Verification items for the finished model (mm, model axes). A direction names the side the tool comes from. Coordinates: 2 decimals unless noted, no trailing zeros. Order: outer loops, then holes, each group sorted by start corner. A loop starts at its lowest first (then second) coordinate and runs counter-clockwise, first axis right, second up. Notation, with made-up numbers: M -8,9 L 31,9 A28 ccw 31,42 Z; hole C 19,72.5 d6. An arc over 180 degrees is marked long. Write item = value, one per line.
```python
from build123d import *

# Parameters (mm, degrees)
BOSS_EXTRUDE1_DEPTH = 1000
CUT_EXTRUDE1_DEPTH  = 3.375
LPATTERN1_COUNT     = 20
LPATTERN1_PITCH     = 50


with BuildPart() as part:
    # Sketch1 → Boss-Extrude1 (new body)
    with BuildSketch(Plane.XY):
        with BuildLine():
            Line((0, 0.3), (0, 20.125))
            ThreePointArc((0, 20.125), (0.02283614, 20.23980503), (0.087867966, 20.337132034))
            Line((0.087867966, 20.337132034), (2.162867966, 22.412132034))
            ThreePointArc((2.162867966, 22.412132034), (2.375, 22.5), (2.587132034, 22.412132034))
            Line((2.587132034, 22.412132034), (4.662132034, 20.337132034))
            ThreePointArc((4.662132034, 20.337132034), (4.72716386, 20.23980503), (4.75, 20.125))
            Line((4.75, 20.125), (4.75, 19.85))
            ThreePointArc((4.75, 19.85), (4.662132034, 19.637867966), (4.45, 19.55))
            Line((4.45, 19.55), (2.375, 19.55))
            Line((2.375, 19.55), (2.375, 0.3))
            ThreePointArc((2.375, 0.3), (2.287132034, 0.087867966), (2.075, 0))
            Line((2.075, 0), (0.3, 0))
            ThreePointArc((0.3, 0), (0.087867966, 0.087867966), (0, 0.3))
        make_face()
    extrude(amount=BOSS_EXTRUDE1_DEPTH)

    # Sketch2 → Cut-Extrude1 (cut, through all)
    with BuildSketch(Plane(origin=(2.375, 0, 0), x_dir=(0, 0, -1), z_dir=(1, 0, 0))):
        with BuildLine():
            Line((-22.35, 12.7), (-22.35, 6))
            ThreePointArc((-22.35, 6), (-25, 3.35), (-27.65, 6))
            Line((-27.65, 6), (-27.65, 12.7))
            ThreePointArc((-27.65, 12.7), (-25, 15.35), (-22.35, 12.7))
        make_face()
    cut_extrude1 = extrude(amount=-CUT_EXTRUDE1_DEPTH, mode=Mode.SUBTRACT)

    # LPattern1: Cut-Extrude1 ×20
    with Locations(*[(0, 0, i * LPATTERN1_PITCH) for i in range(1, LPATTERN1_COUNT)]):
        add(cut_extrude1, mode=Mode.SUBTRACT)


solid = part.part
```
Item 1: Sectioned sample at A-A, the plane z = 299. Enter the section's corners in (x, y) (3 decimals), then the cut area to 3 significant figures.
Report:
outline = M 0,0.3 A0.3 ccw 0.3,0 L 2.075,0 A0.3 ccw 2.375,0.3 L 2.375,19.55 L 4.45,19.55 A0.3 ccw 4.75,19.85 L 4.75,20.125 A0.3 ccw 4.662,20.337 L 2.587,22.412 A0.3 ccw 2.163,22.412 L 0.088,20.337 A0.3 ccw 0,20.125 Z
area = 55.3 mm^2
Item 2: Tool access check on faces 1 (the flat face through (0, 10, 493)), 2 (the flat face through (2.375, 10, 493)). Record the directions out of +Z, -Z, +X, -X, +Y, -Y that give a thin tool (end or side, any length) a straight path to the whole face; none if there is none.
Report:
face_1 = +Z, -Z, -X, +Y, -Y
face_2 = +Z, -Z, +X, -Y
Item 3: Gauge pin test, flat ends, axial feed: pin 1 (2 mm diameter, centred on x = 1, z = 672, fed in from -Y); pin 2 (12 mm diameter, centred on y = 9.5, z = 222, fed in from +X) (3 decimals). Record the tip position at first contact, or that the pin passes through.
Report:
pin_1 = 0
pin_2 = 2.375
Item 4: Scan lines: L1, parallel to X at y = 18.75, z = 92.5 (3 decimals); L2, parallel to X at y = 20.5, z = 523; L3, parallel to Y at x = 1.7, z = 574.5. Record each from-to range of solid material in increasing order. Write a range as from..to.
Report:
L1 = 0..2.375
L2 = 0.25..4.5
L3 = 0..3.4, 15.3..21.95
